Design review of the part shown in the three views and the two pictorial views. Dimensions are in mm from the part's minimum x, y and z. A direction names the side the tool comes from. Round coordinates to 2 decimals unless told otherwise and drop trailing zeros. Write each loop counter-clockwise with the first axis right and the second up, starting at its lowest first coordinate (ties: lowest second). Pieces come first, ordered by that corner, then holes. Notation, with made-up numbers: (64, 84) -> (113, 84) arc R26 ccw to (113, 105) -> close; hole circle Ø6 at (53, 60). An arc over 180 degrees is marked (long way). Return JSON: item names as keys, results as strings. Group by question number.
1. Take a section at B-B, the plane z = 30. Write out the cut boundary in (x, y).
2. Take a section at A-A, the plane y = 2.85. Write out the cut boundary in (x, z) (1 decimal).
3. For line 1 along X through (y, z) = (1.2, 42); line 2 along Y through (x, z) = (7, 40); line 3 along Z through (x, y) = (34, 3.55), list the stretches that pass through material, from the lowest coordinate up. Write a range as from..to.
4. Clearance check with flat-ended pins moving along their axes: P1, Ø2.5, axis at x = 42, z = 3, coming from the +Y side; P2, Ø0.6, axis at x = 19.5, y = 2.5, coming from the +Z side; P3, Ø5, axis at x = 42, z = 42, coming from the +Y side; P4, Ø0.6, axis at y = 3.5, z = 18, coming from the -X side. State where each tip first meets the part, or that it passes through.
5. Tool access review of the marked faces 1 and 2: name each direction out of +Z, -Z, +X, -X, +Y, -Y from which nothing blocks a thin tool from reaching the whole face with its end or side.
6. Take a section at C-C, the plane x = 14. Write out the cut boundary in (y, z).
7. Take a section at D-D, the plane z = 35. Write out the cut boundary in (x, y).
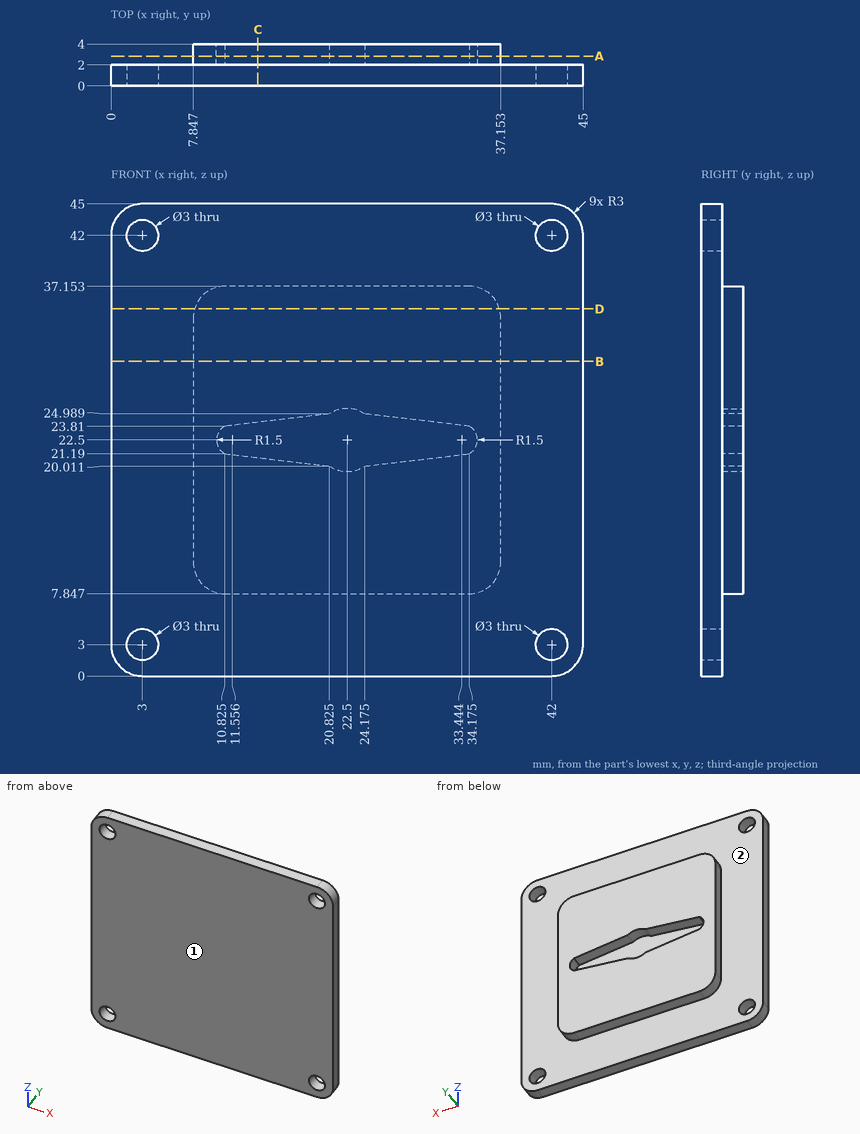
Output:
{
 "1": {"outline": "(0, 0) -> (45, 0) -> (45, 2) -> (37.15, 2) -> (37.15, 4) -> (7.85, 4) -> (7.85, 2) -> (0, 2) -> close"},
 "2": {"outline": "(7.8, 10.8) arc R3 ccw to (10.8, 7.8) -> (34.2, 7.8) arc R3 ccw to (37.2, 10.8) -> (37.2, 34.2) arc R3 ccw to (34.2, 37.2) -> (10.8, 37.2) arc R3 ccw to (7.8, 34.2) -> close; hole (10.8, 21.2) -> (20.8, 20) arc R3 ccw to (24.2, 20) -> (34.2, 21.2) arc R1.5 ccw to (34.2, 23.8) -> (24.2, 25) arc R3 ccw to (20.8, 25) -> (10.8, 23.8) arc R1.5 ccw to start"},
 "3": {"line 1": "x = 0..1.5, 4.5..40.5, 43.5..45", "line 2": "y = 0..2", "line 3": "z = 7.85..21.17, 23.83..37.15"},
 "4": {"P1": "passes through", "P2": "stops at z = 37.15", "P3": "stops at y = 2", "P4": "stops at x = 7.85"},
 "5": {"face 1": "+Z, -Z, +X, -X, -Y", "face 2": "+Y"},
 "6": {"outline": "(0, 0) -> (2, 0) -> (2, 7.85) -> (4, 7.85) -> (4, 20.82) -> (2, 20.82) -> (2, 24.18) -> (4, 24.18) -> (4, 37.15) -> (2, 37.15) -> (2, 45) -> (0, 45) -> close"},
 "7": {"outline": "(0, 0) -> (45, 0) -> (45, 2) -> (37.03, 2) -> (37.03, 4) -> (7.97, 4) -> (7.97, 2) -> (0, 2) -> close"}
}
